Here's the drawing with two shaded views (mm, measured from the low corner). I have some questions. A direction names the side the tool comes from. Round coordinates to 2 decimals unless told otherwise and drop trailing zeros. Loops run counter-clockwise (first coordinate to the right, second up) from the corner with the lowest first, then second, coordinate; pieces in that order, holes last.
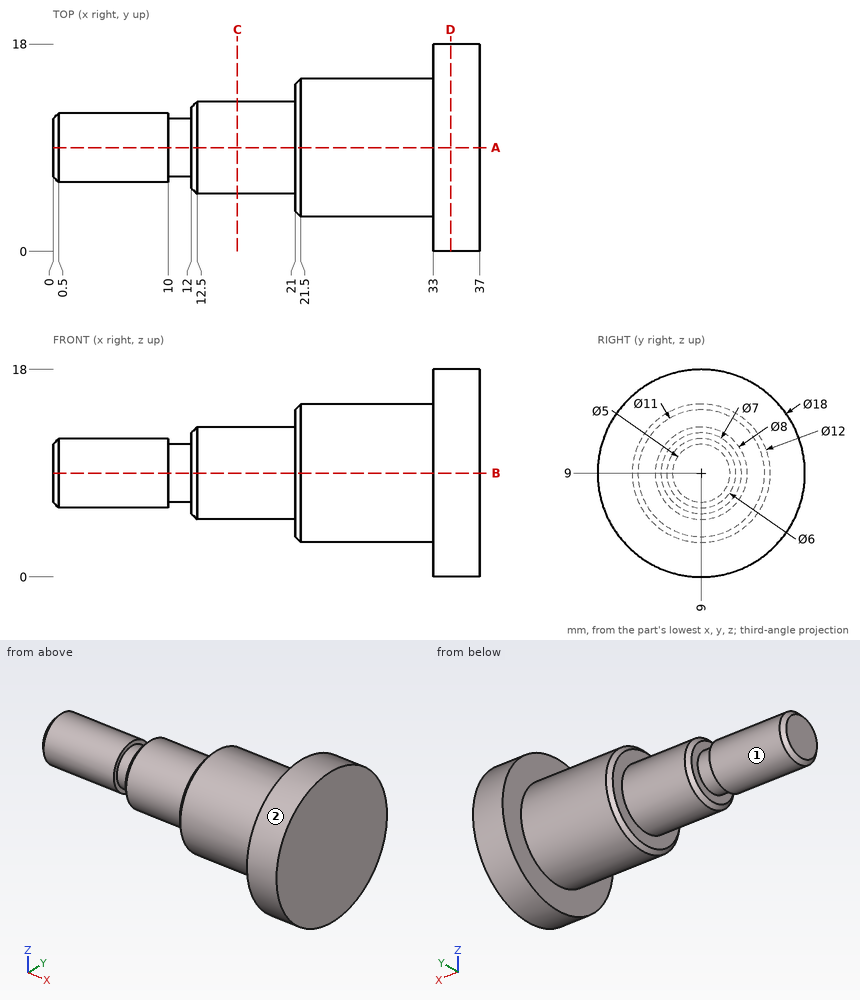
(1) For the marked faces 1 and 2, which set-ups out of +Z, -Z, +X, -X, +Y, -Y let a thin tool reach every point of the face, with its end or its side?
Worked answers:
face 1: -X
face 2: +X, -X
(2) Will these pins go through, and if not, where does the flat tip stop? P1, Ø10, axis at x = 28.5, y = 7, coming from the +Z side; P2, Ø2, axis at x = 21, z = 14.5, coming from the +Y side; P3, Ø8, axis at x = 24.5, y = 12.5, coming from the +Z side; P4, Ø1.5, axis at x = 21, y = 14, coming from the +Z side.
Worked answers:
P1: stops at z = 18
P2: stops at y = 12.81
P3: stops at z = 15
P4: stops at z = 13.03
(3) If we section it at A-A, the plane y = 9: List the corners of the cut face in (x, z) for me, then the cut area to 3 significant figures.
Worked answers:
outline: (0, 6.5) - (0.5, 6) - (10, 6) - (10, 6.5) - (12, 6.5) - (12, 5.5) - (12.5, 5) - (21, 5) - (21, 3.5) - (21.5, 3) - (33, 3) - (33, 0) - (37, 0) - (37, 18) - (33, 18) - (33, 15) - (21.5, 15) - (21, 14.5) - (21, 13) - (12.5, 13) - (12, 12.5) - (12, 11.5) - (10, 11.5) - (10, 12) - (0.5, 12) - (0, 11.5) - close
area: 357 mm2
(4) If we section it at C-C, the plane x = 16: List the corners of the cut face in (y, z) for me, then the cut area to 3 significant figures.
Worked answers:
outline: circle Ø8 at (9, 9)
area: 50.3 mm2
(5) If I drill on line 1 (X direction, y = 8.5, z = 2.25); line 2 (Y direction, x = 22.5, z = 8.75); line 3 (X direction, y = 10.5, z = 4), over which ranges is the centre line in solid material (lowest first)?
Worked answers:
line 1: x = 33 to 37
line 2: y = 3.01 to 14.99
line 3: x = 21 to 37
(6) If we section it at D-D, the plane x = 34.5: List the corners of the cut face in (y, z) for me.
Worked answers:
outline: circle Ø18 at (9, 9)
